Check sheet for the modelled part. Datum: model origin and axes. Units: mm. Coordinates: 2 decimals unless noted, no trailing zeros. Loops run counter-clockwise (first coordinate to the right, second up) from the corner with the lowest first, then second, coordinate; pieces in that order, holes last. Notation, with made-up numbers: (34.25, 26) - (81.25, 26) arc R29 cw to (81.25, 48) - close; hole circle Ø3 at (46.25, -29.75). An arc over 180 degrees is marked (long way). Write each question's results on one line, items separated by ' | '. Start each with the question number.
1. Cross-section at A-A (z = -30.5). Record the cut outline in (x, y), and give its area (3 significant figures).
2. Cross-section at C-C (y = 0.1). Record the cut outline in (x, z).
3. Gauge pin test, flat ends, axial feed: P1, Ø1.8, axis at x = 78.5, z = 104.5, coming from the -Y side; P2, Ø2.5, axis at x = -78.37, z = -104.6, coming from the -Y side. Record the tip position at first contact, or that the pin passes through.
4. Thickness scan on line 1 (Z direction, x = -78.5, y = 0.3); line 2 (Z direction, x = 78.5, y = 0.1); line 3 (Z direction, x = -44, y = 0.25). Record the ranges inside material, lowest first. Write a range as [from, to].
5. Cross-section at B-B (x = -50). Record the cut outline in (y, z), and give its area (3 significant figures).
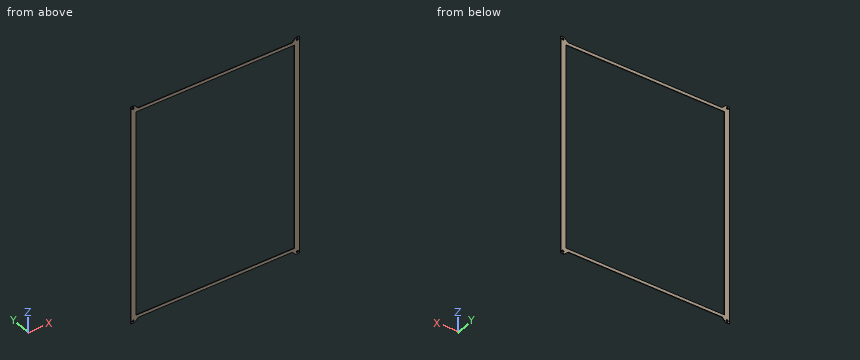
```python
from build123d import *

# Parameters (mm, degrees)
CROQUIS1_R              = 1
CROQUIS1_W              = 151
CROQUIS1_H              = 200
SALIENTE_EXTRUIR1_DEPTH = 0.5


with BuildPart() as part:
    # Croquis1 → Saliente-Extruir1 (new body)
    with BuildSketch(Plane(origin=(0, 0, 0), x_dir=(1, 0, 0), z_dir=(0, 1, 0))):
        Polygon((-80.5, -106.4), (-80.5, -106.5), (-80.4, -106.5), (-76.9, -106.5), (-73.4, -103), (73.5, -103), (77, -106.5), (80.5, -106.5), (80.5, 106.5), (77, 106.5), (73.5, 103), (-73.4, 103), (-76.9, 106.5), (-80.5, 106.5), align=None)
        with Locations((-78.5, -104.5)):
            Circle(CROQUIS1_R, mode=Mode.SUBTRACT)
        with Locations((78.5, -104.5)):
            Circle(CROQUIS1_R, mode=Mode.SUBTRACT)
        with Locations((78.629753046, 104.40240388)):
            Circle(CROQUIS1_R, mode=Mode.SUBTRACT)
        with Locations((-78.370125817, 104.597434861)):
            Circle(CROQUIS1_R, mode=Mode.SUBTRACT)
        Rectangle(CROQUIS1_W, CROQUIS1_H, mode=Mode.SUBTRACT)
    extrude(amount=SALIENTE_EXTRUIR1_DEPTH)


solid = part.part
```
Established:
1) outline: (-80.5, 0) - (-75.5, 0) - (-75.5, 0.5) - (-80.5, 0.5) - close; (75.5, 0) - (80.5, 0) - (80.5, 0.5) - (75.5, 0.5) - close | area: 5.00 mm^2
2) outline: (-80.5, -106.5) - (-76.9, -106.5) - (-73.4, -103) - (73.5, -103) - (77, -106.5) - (80.5, -106.5) - (80.5, 106.5) - (77, 106.5) - (73.5, 103) - (-73.4, 103) - (-76.9, 106.5) - (-80.5, 106.5) - close; hole circle Ø2 at (-78.5, 104.5); hole circle Ø2 at (-78.37, -104.6); hole (-75.5, -100) - (75.5, -100) - (75.5, 100) - (-75.5, 100) - close; hole circle Ø2 at (78.5, 104.5); hole circle Ø2 at (78.63, -104.4)
3) P1: through | P2: y = 0
4) line 1: [-106.5, -105.59], [-103.61, 103.5], [105.5, 106.5] | line 2: [-106.5, -105.39], [-103.41, 103.5], [105.5, 106.5] | line 3: [-103, -100], [100, 103]
5) outline: (0, -103) - (0.5, -103) - (0.5, -100) - (0, -100) - close; (0, 100) - (0.5, 100) - (0.5, 103) - (0, 103) - close | area: 3.00 mm^2
